```python
from build123d import *

# Parameters (mm, degrees)
BOX002_W          = 5
BOX002_H          = 20
BOX002_DEPTH      = 7.6
BOX001_W          = 15
BOX001_H          = 26.3
BOX001_DEPTH      = 15.1
CYLINDER_R        = 3
CYLINDER_DEPTH    = 5.3
CYLINDER001_R     = 3
CYLINDER001_DEPTH = 5.3
BOX_W             = 47
BOX_H             = 26.3
BOX_DEPTH         = 11


with BuildPart() as plugs:
    # Box002 → Box002 (new body)
    with BuildSketch(Plane(origin=(42, 3.35, 1), x_dir=(1, 0, 0), z_dir=(0, 0, 1))):
        with Locations((2.5, 10)):
            Rectangle(BOX002_W, BOX002_H)
    extrude(amount=BOX002_DEPTH)


with BuildPart() as cube001:
    # Box001 → Box001 (new body)
    with BuildSketch(Plane(origin=(32, 0, 0), x_dir=(1, 0, 0), z_dir=(0, 0, 1))):
        with Locations((7.5, 13.15)):
            Rectangle(BOX001_W, BOX001_H)
    extrude(amount=BOX001_DEPTH)


with BuildPart() as cylinder:
    # Cylinder → Cylinder (new body)
    with BuildSketch(Plane(origin=(0, 4, 3), x_dir=(0, 0, 1), z_dir=(-1, 0, 0))):
        Circle(CYLINDER_R)
    extrude(amount=CYLINDER_DEPTH)


with BuildPart() as cylinder001:
    # Cylinder001 → Cylinder001 (new body)
    with BuildSketch(Plane(origin=(0, 22, 3), x_dir=(0, 0, 1), z_dir=(-1, 0, 0))):
        Circle(CYLINDER001_R)
    extrude(amount=CYLINDER001_DEPTH)


with BuildPart() as receiver_model:
    # Box → Box (new body)
    with BuildSketch(Plane.XY):
        with Locations((23.5, 13.15)):
            Rectangle(BOX_W, BOX_H)
    extrude(amount=BOX_DEPTH)

    # Fusion: union Cube001, Cylinder, Cylinder001
    add(cube001.part)
    add(cylinder.part)
    add(cylinder001.part)

    # Cut: cut Plugs
    add(plugs.part, mode=Mode.SUBTRACT)


solid = receiver_model.part
```
Work out the finished part from the listing and answer in its coordinate system (mm). A direction names the side the tool comes from. Give positions to 0.01 mm unless a question says otherwise; leave off trailing zeros. Order: outer loops, then holes, each group sorted by start corner. A loop starts at its lowest first (then second) coordinate and runs counter-clockwise, first axis right, second up. Notation, with made-up numbers: (-15, 63) -> (25, 63) arc R21 ccw to (25, 78) -> close; hole circle Ø1 at (-36, 21). An arc over 180 degrees is marked (long way). Answer as CSV lines item,"result". Start each with the question number.
(1) Section A-A, the plane z = 6.75 is taken. Write down the section's boundary in (x, y), plus the area to 3 significant figures.
(2) Consider line 1 along Y through (x, z) = (43, 3.75); line 2 along Z through (x, y) = (24, 21.25); line 3 along X through (y, z) = (17.25, 1.75). Determine where each line is inside the solid, lowest interval first.
(3) Each of these flat-tipped pins is pushed along its axis until it touches: pin 1 Ø6 at (x, z) = (19.5, 2.5) entering from -Y; pin 2 Ø13 at (x, y) = (17.5, 18.5) entering from +Z; pin 3 Ø4 at (y, z) = (16.5, 4) entering from +X; pin 4 Ø1.2 at (y, z) = (9.5, 13.5) entering from -X. Where does it stop, or does it pass through?
(4) For a pull along Z with two mould halves and no side action, classify faces 1 (the flat face through (44, 13, 1)), 2 (the flat face through (-5.3, 4, 3)), 3 (the flat face through (44, 13, 8.6)), 4 (the flat face through (39, 13, 15.1)) as released by +Z, released by -Z, zero draft, split by the parting line, or undercut.
(5) Which of the six approach directions +Z, -Z, +X, -X, +Y, -Y give full straight-line access (tool end or side, diameter ignored) to faces 5 (the flat face through (23, 13, 0)), 6 (the flat face through (44, 23.35, 5)), 7 (the cylindrical face through (-2.6, 2.2, 0.6)), 8 (the flat face through (16, 13, 11)), 9 (the flat face through (23, 26.3, 6))?
(6) Section C-C, the plane y = 16 is taken. Write down the section's boundary in (x, z), plus the area to 4 significant figures.
(7) Section D-D, the plane z = 3 is taken. Write down the section's boundary in (x, y), plus the area to 3 significant figures.
(8) Section B-B, the plane x = 42.5 is taken. Write down the section's boundary in (y, z), plus the area to 3 significant figures.
Entries:
1,outline,"(0, 0) -> (47, 0) -> (47, 3.35) -> (42, 3.35) -> (42, 23.35) -> (47, 23.35) -> (47, 26.3) -> (0, 26.3) -> close"
1,area,"1,140 mm²"
2,line 1,"0 to 3.35, 23.35 to 26.3"
2,line 2,"0 to 11"
2,line 3,"0 to 42"
3,pin 1,"y = 0"
3,pin 2,"z = 11"
3,pin 3,"x = 42"
3,pin 4,"x = 32"
4,face 1,"undercut"
4,face 2,"zero draft"
4,face 3,"undercut"
4,face 4,"released by +Z"
5,face 5,"-Z, +X, -X, +Y, -Y"
5,face 6,"+X"
5,face 7,"-X"
5,face 8,"+Z, -X, +Y, -Y"
5,face 9,"+Z, -Z, +X, -X, +Y"
6,outline,"(0, 0) -> (47, 0) -> (47, 1) -> (42, 1) -> (42, 8.6) -> (47, 8.6) -> (47, 15.1) -> (32, 15.1) -> (32, 11) -> (0, 11) -> close"
6,area,"540.5 mm²"
7,outline,"(-5.3, 1) -> (0, 1) -> (0, 0) -> (47, 0) -> (47, 3.35) -> (42, 3.35) -> (42, 23.35) -> (47, 23.35) -> (47, 26.3) -> (0, 26.3) -> (0, 25) -> (-5.3, 25) -> (-5.3, 19) -> (0, 19) -> (0, 7) -> (-5.3, 7) -> close"
7,area,"1,200 mm²"
8,outline,"(0, 0) -> (26.3, 0) -> (26.3, 15.1) -> (0, 15.1) -> close; hole (3.35, 1) -> (23.35, 1) -> (23.35, 8.6) -> (3.35, 8.6) -> close"
8,area,"245 mm²"
